Autodesk Inventor part; units mm, degrees
ref_plane "Work Plane1" through (6, 0, 0) normal (1, 0, 0) x (0, 0, -1)
ref_plane "Work Plane2" through (6, 0, 0) normal (-1, 0, 0) x (0, 0, 1)
ref_plane "YZ Plane" through (0, 0, 0) normal (1, 0, 0) x (0, 1, 0)
sketch "Sketch2" plane through (0, 0, 0) normal (1, 0, 0) x (0, 1, 0)
  line L0 (0, 0) -> (15, 0)
  line L1 (15, 0) -> (15, -10)
  line L2 (15, -10) -> (0, -10)
  line L3 (0, -10) -> (0, 0)
  dimension "d4" = 15
  dimension "d5" = 10
extrude "Extrusion2" add sketch "Sketch2" along normal blind 12
sketch "Sketch3" plane through (0, 0, 0) normal (0, 0, 1) x (1, 0, 0)
  line L0 (0, 0) -> (1, 0)
  line L1 (0, 0) -> (12, 0)
  line L2 (1, 0) -> (1, 13.5)
  line L3 (1, 13.5) -> (11, 13.5)
  line L4 (11, 13.5) -> (11, 0)
  line L5 (11, 0) -> (1, 0)
  dimension "d8" = 1
  dimension "d9" = 13.5
  dimension "d10" = 10
extrude "Extrusion3" cut sketch "Sketch3" against normal blind 8
sketch "Sketch4" plane through (0, 0, -10) normal (0, 0, -1) x (-1, 0, 0)
  line L0 (0, 15) -> (-12, 15)
  line L1 (0, 0) -> (-12, 0)
  line L2 (-12, 15) -> (0, 15)
  line L3 (0, 15) -> (0, 0)
  line L4 (0, 0) -> (-12, 0)
  line L5 (-12, 0) -> (-12, 15)
extrude "Extrusion4" add sketch "Sketch4" along normal blind 2
sketch "Sketch5" plane through (0, 0, -8) normal (0, 0, 1) x (1, 0, 0)
  line L0 (1, 13.5) -> (11, 13.5)
  line L1 (6, 13.5) -> (6, 10)
  line L2 (6, 10) -> (6, 3.5)
  circle A0 centre (6, 10) radius 1.2295
  circle A1 centre (6, 3.5) radius 1.2295
  point P0 (0, 0)
  dimension "d15" = 3.5
  dimension "d16" = 6.5
  dimension "d17" = 2.459
  dimension "d18" = 2.459
extrude "Extrusion5" cut sketch "Sketch5" against normal blind 4
sketch "Sketch6" plane through (0, 0, -8) normal (0, 0, 1) x (1, 0, 0)
  circle A0 centre (6, 10) radius 1.2295
  circle A1 centre (6, 10) radius 2.7
  circle A2 centre (6, 3.5) radius 1.2295
  circle A3 centre (6, 3.5) radius 2.7
  point P0 (0, 0)
  dimension "d21" = 5.4
  dimension "d22" = 5.4
extrude "Extrusion6" cut sketch "Sketch6" against normal blind 1.1
sketch "Sketch15" plane through (12, 0, 0) normal (1, 0, 0) x (0, 0, -1)
  line L0 (0, 15) -> (12, 15)
  line L1 (12, 15) -> (12, 0)
  line L2 (0, 15) -> (12, 15)
  line L3 (12, 15) -> (12, 0)
  line L4 (12, 0) -> (0, 0)
  line L5 (0, 0) -> (0, 15)
extrude "Extrusion14" add sketch "Sketch15" along normal blind 4
ref_plane "Work Plane1" through (6, 0, 0) normal (1, 0, 0) x (0, 0, -1)
mirror "Mirror1" about plane through (6, 0, 0) normal (1, 0, 0) of "Extrusion14"
sketch "Sketch16" plane through (1, 0, -8) normal (0, -1, 0) x (1, 0, 0)
  line L0 (10, 0) -> (0, 0)
  line L1 (5, 0) -> (7.5, 0)
  line L2 (7.5, 0) -> (7.5, -4)
  line L3 (-5, -4) -> (15, -4)
  line L4 (7.5, -4) -> (2.5, -4)
  line L5 (2.5, -4) -> (2.5, 0)
  line L6 (2.5, 0) -> (5, 0)
  point P0 (-1, 8)
  dimension "d61" = 2.5
  dimension "d62" = 4
  dimension "d63" = 5
  dimension "d64" = 4
extrude "Extrusion15" add sketch "Sketch16" along normal blind 10
sketch "Sketch18" plane through (0, 0, -12) normal (0, 0, -1) x (-1, 0, 0)
  line L0 (-16, 15) -> (4, 15)
  line L1 (4, 0) -> (-3.5, 0)
  line L2 (-16, 15) -> (4, 15)
  line L3 (4, 15) -> (4, 0)
  line L4 (4, 0) -> (-16, 0)
  line L5 (-16, 0) -> (-16, 15)
  line L6 (-8.5, -10) -> (-3.5, -10)
  line L7 (-3.5, 0) -> (-8.5, 0)
  line L8 (-8.5, 0) -> (-8.5, -10)
  line L9 (-8.5, -10) -> (-3.5, -10)
  line L10 (-3.5, -10) -> (-3.5, 0)
  circle A0 centre (-6, 3.5) radius 1.2295
  circle A1 centre (-6, 3.5) radius 1.2295
  circle A2 centre (-6, 10) radius 1.2295
  circle A3 centre (-6, 10) radius 1.2295
  point P0 (0, 0)
extrude "Extrusion16" add sketch "Sketch18" along normal blind 1
sketch "Sketch19" plane through (16, 0, 0) normal (1, 0, 0) x (0, 0, -1)
  line L0 (0, 15) -> (13, 15)
  line L1 (0, 15) -> (0, 40)
  line L2 (-5, 45) -> (-12, 45)
  line L3 (13, 45) -> (13, 15)
  line L4 (0, 57) -> (-12, 57)
  line L5 (0, 57) -> (13, 45)
  line L6 (-9, 51) -> (-12, 57)
  line L7 (-9, 51) -> (-12, 45)
  arc A0 (0, 40) -> (-5, 45) centre (-5, 40) ccw
  point P0 (0, 0)
  point P1 (0, 45)
  dimension "d69" = 30
  dimension "d75" = 5
extrude "Extrusion17" add sketch "Sketch19" against normal blind 20
sketch "Sketch20" plane through (0, 0, -13) normal (0, 0, -1) x (-1, 0, 0)
  circle A0 centre (-6, 10) radius 1.2295
  circle A1 centre (-6, 10) radius 1.925
  circle A2 centre (-6, 3.5) radius 1.2295
  circle A3 centre (-6, 3.5) radius 1.925
  point P0 (0, 0)
  dimension "d80" = 3.85
  dimension "d81" = 3.85
extrude "Extrusion18" cut sketch "Sketch20" against normal blind 10
sketch "Sketch22" plane through (16, 0, 0) normal (1, 0, 0) x (0, 0, -1)
  line L0 (0, 57) -> (-12, 57)
  line L1 (-12, 57) -> (0, 57)
  line L2 (13, 45) -> (0, 57)
  line L3 (0, 57) -> (13, 45)
  line L4 (13, 0) -> (13, 45)
  line L5 (13, 45) -> (13, 0)
  line L6 (0, 0) -> (8, 0)
  line L7 (13, 0) -> (0, 0)
  line L8 (0, 40) -> (0, 0)
  line L9 (0, 0) -> (0, 40)
  line L10 (-12, 45) -> (-5, 45)
  line L11 (-5, 45) -> (-12, 45)
  line L12 (-12, 45) -> (-9, 51)
  line L13 (-12, 45) -> (-9, 51)
  line L14 (-12, 57) -> (-9, 51)
  line L15 (-9, 51) -> (-12, 57)
  arc A0 (0, 40) -> (-5, 45) centre (-5, 40) ccw
extrude "Extrusion20" cut sketch "Sketch22" against normal blind 1.75
ref_plane "Work Plane2" through (6, 0, 0) normal (-1, 0, 0) x (0, 0, 1)
mirror "Mirror2" about plane through (6, 0, 0) normal (-1, 0, 0) of "Extrusion20"
properties part number "3point finger"
The listing builds one solid part. Answer for the finished solid, in the listing's coordinates (mm). A direction names the side the tool comes from. Round coordinates to 2 decimals unless told otherwise and drop trailing zeros. Order: outer loops, then holes, each group sorted by start corner. A loop starts at its lowest first (then second) coordinate and runs counter-clockwise, first axis right, second up. Notation, with made-up numbers: (37.5, 78) -> (87.5, 78) arc R9 ccw to (87.5, 94) -> close; hole circle Ø7 at (53, 9.5). An arc over 180 degrees is marked (long way). Write each question's results on one line, items separated by ' | '. Start each with the question number.
Q1. Find section C-C (x = -0.25). Determine the outline of the cut face in (y, z), then the cut area to 3 significant figures.
Q2. Which of the six approach directions +Z, -Z, +X, -X, +Y, -Y give full straight-line access (tool end or side, diameter ignored) to faces 4 (the flat face through (6, 24, 0)), 5 (the flat face through (6, -1, -8)), 6 (the flat face through (6.1, 48, 10.5)), 7 (the flat face through (12, 0, -8)), 8 (the flat face through (3.5, -5, -11))?
Q3. Find section D-D (z = -0.75). Determine the outline of the cut face in (x, y).
Q4. Find section B-B (x = 6). Determine the outline of the cut face in (y, z) (3 decimals).
Q5. Straight lines are drawn through the part: probe 1 along Y at (x, z) = (6, -10) (3 decimals); probe 2 along Y at (x, z) = (6, -8.3); probe 3 along Z at (x, y) = (11.5, 29). For each, find the intervals that lie inside material, in ascending order. Write a range as from..to.
Q6. The mould has two halves that part along Y. Classify faces 1 (the flat face through (6, 24, -13)), 2 (the cylindrical face through (7.923, 3.585, -11.077)), 3 (the flat face through (6, -10, -10)): pulls with the +Y half, pulls with the -Y half, needs draft (parallel to the pull), parting line crosses it, or undercut.
Q7. Each of these flat-tipped pins is pushed along its axis until it touches: pin 1 (1.5 mm diameter, centred on x = 11, y = 47, fed in from +Z) (3 decimals); pin 2 (5.5 mm diameter, centred on x = 3.5, z = 10, fed in from -Y); pin 3 (1.6 mm diameter, centred on x = 6.5, y = 11.5, fed in from +Z). Where does it stop, or does it pass through?
Q8. Find section A-A (y = 3.5). Determine the outline of the cut face in (x, z) (3 decimals), then the cut area to 3 significant figures.
Worked answers:
1) outline: (0, -13) -> (45, -13) -> (57, 0) -> (57, 12) -> (51, 9) -> (45, 12) -> (45, 5) arc R5 cw to (40, 0) -> (0, 0) -> close | area: 794 mm2
2) face 4: +Z, +X, -X, -Y | face 5: +Z, -Y | face 6: +Z, +X, -X | face 7: +Z, -Z, +X, -Y | face 8: +Z, -Z, -X, -Y
3) outline: (-2.25, 0) -> (1, 0) -> (1, 13.5) -> (11, 13.5) -> (11, 0) -> (14.25, 0) -> (14.25, 56.31) -> (-2.25, 56.31) -> close
4) outline: (-10, -13) -> (1.575, -13) -> (1.575, -9.1) -> (0.8, -9.1) -> (0.8, -8) -> (-10, -8) -> close; (5.425, -13) -> (8.075, -13) -> (8.075, -9.1) -> (7.3, -9.1) -> (7.3, -8) -> (6.2, -8) -> (6.2, -9.1) -> (5.425, -9.1) -> close; (11.925, -13) -> (45, -13) -> (57, 0) -> (57, 12) -> (51, 9) -> (45, 12) -> (45, 5) arc R5 cw to (40, 0) -> (13.5, 0) -> (13.5, -8) -> (12.7, -8) -> (12.7, -9.1) -> (11.925, -9.1) -> close
5) probe 1: y = -10..1.575, 5.425..8.075, 11.925..47.769 | probe 2: y = -10..0.8, 6.2..7.3, 12.7..49.34 | probe 3: z = -13..0
6) face 1: needs draft | face 2: undercut | face 3: pulls with the -Y half
7) pin 1: stops at z = 11.375 | pin 2: stops at y = 45 | pin 3: stops at z = -9.1
8) outline: (-2.25, -13) -> (4.075, -13) -> (4.075, -9.1) -> (3.3, -9.1) -> (3.3, -8) -> (1, -8) -> (1, 0) -> (-2.25, 0) -> close; (7.925, -13) -> (14.25, -13) -> (14.25, 0) -> (11, 0) -> (11, -8) -> (8.7, -8) -> (8.7, -9.1) -> (7.925, -9.1) -> close | area: 114 mm2
